Autodesk Inventor part; units mm, degrees
ref_plane "YZ Plane" through (0, 0, 0) normal (1, 0, 0) x (0, 1, 0)
ref_plane "XZ Plane" through (0, 0, 0) normal (0, 1, 0) x (-1, 0, 0)
ref_plane "XY Plane" through (0, 0, 0) normal (0, 0, 1) x (1, 0, 0)
ref_plane "작업 평면1" through (-67, 45, 0) normal (0, 0, 1) x (1, 0, 0)
sketch "스케치1" plane through (-67, 45, 0) normal (0, 0, 1) x (1, 0, 0)
  line L0 (0, 0) -> (70, 0)
  line L1 (70, 0) -> (70, 6)
  line L2 (0, 6) -> (70, 6)
  line L3 (0, 0) -> (0, 6)
  line L4 (70, 0) -> (64, 0)
  line L5 (64, 0) -> (64, -90)
  line L6 (64, -90) -> (70, -90)
  line L7 (70, -90) -> (70, 0)
  line L8 (70, -90) -> (0, -90)
  line L9 (0, -90) -> (0, -96)
  line L10 (70, -96) -> (0, -96)
  line L11 (70, -90) -> (70, -96)
  line L12 (70, 6) -> (0, 6)
  line L13 (0, 6) -> (0, -96)
  line L14 (0, -96) -> (70, -96)
  line L15 (70, -96) -> (70, 6)
  point P0 (67, -45)
extrude "돌출1" add sketch "스케치1" along normal blind 6
sketch "스케치2" plane through (-67, 45, 6) normal (0, 0, 1) x (1, 0, 0)
  circle A0 centre (6, -8) radius 1.25
  circle A1 centre (14, -8) radius 1.25
  line L0 (20, -3) -> (0, -3)
  line L1 (20, -3) -> (20, -13)
  line L2 (0, -13) -> (20, -13)
  line L3 (0, -3) -> (0, -13)
  circle A2 centre (57.5, -8) radius 1.25
  line L4 (61, -13) -> (61, -3)
  line L5 (54, -13) -> (61, -13)
  line L6 (54, -3) -> (54, -13)
  line L7 (61, -3) -> (54, -3)
  circle A3 centre (56, -83.5) radius 1.25
  line L8 (51, -87) -> (61, -87)
  line L9 (51, -80) -> (51, -87)
  line L10 (61, -80) -> (51, -80)
  line L11 (61, -87) -> (61, -80)
  circle A4 centre (14, -82) radius 1.25
  circle A5 centre (6, -82) radius 1.25
  line L12 (0, -87) -> (20, -87)
  line L13 (0, -87) -> (0, -77)
  line L14 (20, -77) -> (0, -77)
  line L15 (20, -87) -> (20, -77)
  point P0 (67, -45)
extrude "돌출2" cut sketch "스케치2" against normal blind 6 contours A0 | A1 | A2 | A3 | A4 | A5
sketch "스케치3" plane through (-67, 45, 6) normal (0, 0, 1) x (1, 0, 0)
  circle A0 centre (57.5, -8) radius 1.25
  circle A1 centre (6, -82) radius 1.25
  circle A2 centre (14, -8) radius 1.25
  circle A3 centre (56, -83.5) radius 1.25
  circle A4 centre (14, -82) radius 1.25
  circle A5 centre (6, -8) radius 1.25
  line L0 (0, 6) -> (0, -96)
  line L1 (0, -96) -> (70, -96)
  line L2 (70, -96) -> (70, 6)
  line L3 (70, 6) -> (0, 6)
  line L4 (70, -96) -> (70, 6)
  line L5 (0, 6) -> (0, -96)
  line L6 (0, -96) -> (70, -96)
  line L7 (70, 6) -> (0, 6)
  line L8 (20, -78) -> (50, -78)
  line L9 (50, -78) -> (50, -12)
  line L10 (50, -12) -> (20, -12)
  line L11 (20, -12) -> (20, -78)
  point P0 (67, -45)
  point P1 (50, -64.8252)
  point P2 (20, -61.3274)
  point P3 (30.9806, -78)
  point P4 (28.8515, -12)
  point P5 (28.8515, -12)
  dimension "d4" = 20
  dimension "d5" = 20
  dimension "d6" = 18
  dimension "d7" = 18
extrude "돌출3" cut sketch "스케치3" against normal blind 6 contours L11 L10 L9 L8
fillet "모깎기1" radius 2 4 edges at (-47, -33, 3) (-17, -33, 3) (-47, 33, 3) (-17, 33, 3)
properties part number "62" material "아크릴, 선명"
Can you work these out from the model? Positions are in its coordinate system, mm. A direction names the side the tool comes from. Give positions to 0.01 mm unless a question says otherwise; leave off trailing zeros. Loops run counter-clockwise (first coordinate to the right, second up) from the corner with the lowest first, then second, coordinate; pieces in that order, holes last. Notation, with made-up numbers: (57, -19.75) -> (97, -19.75) arc R17 cw to (97, -13.75) -> close; hole circle Ø3 at (65, 21.25). An arc over 180 degrees is marked (long way). Use one line per item in the form item = value.
1) If we section it at C-C (y = 25): Please give me the cut outline in (x, z), plus the area to 3 significant figures.
Answers:
outline = (-67, 0) -> (-47, 0) -> (-47, 6) -> (-67, 6) -> close; (-17, 0) -> (3, 0) -> (3, 6) -> (-17, 6) -> close
area = 240 mm²
2) I need wall thicknesses on line 1 along Y through (x, z) = (-61, 1.55); line 2 along Y through (x, z) = (-23.5, 1.3); line 3 along X through (y, z) = (4.5, 0.8). Which ranges of each line are inside material? Lowest first, please.
Answers:
line_1 = -51 to -38.25, -35.75 to 35.75, 38.25 to 51
line_2 = -51 to -33, 33 to 51
line_3 = -67 to -47, -17 to 3
3) If we section it at B-B (z = 3.55): Please give me the cut outline in (x, y).
Answers:
outline = (-67, -51) -> (3, -51) -> (3, 51) -> (-67, 51) -> close; hole circle Ø2.5 at (-61, -37); hole circle Ø2.5 at (-61, 37); hole circle Ø2.5 at (-53, -37); hole circle Ø2.5 at (-53, 37); hole (-47, -31) arc R2 ccw to (-45, -33) -> (-19, -33) arc R2 ccw to (-17, -31) -> (-17, 31) arc R2 ccw to (-19, 33) -> (-45, 33) arc R2 ccw to (-47, 31) -> close; hole circle Ø2.5 at (-11, -38.5); hole circle Ø2.5 at (-9.5, 37)
4) If we section it at D-D (x = -26): Please give me the cut outline in (y, z), plus the area to 3 significant figures.
Answers:
outline = (-51, 0) -> (-33, 0) -> (-33, 6) -> (-51, 6) -> close; (33, 0) -> (51, 0) -> (51, 6) -> (33, 6) -> close
area = 216 mm²
5) For faces 4 (the face through (-67, -1, 3)), 5 (the face through (-47, 0, 3)), which set-ups out of +Z, -Z, +X, -X, +Y, -Y let a thin tool reach every point of the face, with its end or its side?
Answers:
face_4 = +Z, -Z, -X, +Y, -Y
face_5 = +Z, -Z
6) We'd pull the mould along X, two halves only. Please class faces 1 (the face through (3, -1, 3)), 2 (the face through (-46.4, -32.43, 2.96)), 3 (the face through (-48, 1, 0)): released by +X, released by -X, zero draft, split by the parting line, or undercut.
Answers:
face_1 = released by +X
face_2 = undercut
face_3 = zero draft
7) If we section it at A-A (x = -53): Please give me the cut outline in (y, z), plus the area to 3 significant figures.
Answers:
outline = (-51, 0) -> (-38.25, 0) -> (-38.25, 6) -> (-51, 6) -> close; (-35.75, 0) -> (35.75, 0) -> (35.75, 6) -> (-35.75, 6) -> close; (38.25, 0) -> (51, 0) -> (51, 6) -> (38.25, 6) -> close
area = 582 mm²
8) Will this pin go through, and if not, where does the flat tip stop? pin 1 (2 mm diameter, centred on x = -11, y = -38.5, fed in from +Z) (3 decimals).
Answers:
pin_1 = through
